Can you work these out from the model? Positions are in its coordinate system, mm. A direction names the side the tool comes from. Round coordinates to 2 decimals unless told otherwise and drop trailing zeros. Loops run counter-clockwise (first coordinate to the right, second up) from the corner with the lowest first, then second, coordinate; pieces in that order, holes last. Notation, with made-up numbers: (-19.5, -25.5) -> (-9.5, -25.5) arc R19 ccw to (-9.5, -21.5) -> close; hole circle Ø7 at (36.25, 80.5). An arc over 180 degrees is marked (long way). Use a Markdown table: item, result.
from build123d import *

# Parameters (mm, degrees)
SKETCH1_R           = 60
BOSS_EXTRUDE1_DEPTH = 10
SKETCH2_R           = 60
SKETCH2_R_2         = 55
BOSS_EXTRUDE2_DEPTH = 20
SKETCH3_R           = 12.5
CUT_EXTRUDE1_DEPTH  = 11


with BuildPart() as part:
    # Sketch1 → Boss-Extrude1 (new body)
    with BuildSketch(Plane(origin=(0, 0, 0), x_dir=(0, 0, -1), z_dir=(1, 0, 0))):
        Circle(SKETCH1_R)
    extrude(amount=BOSS_EXTRUDE1_DEPTH)

    # Sketch2 → Boss-Extrude2 (add)
    with BuildSketch(Plane(origin=(10, 0, 0), x_dir=(0, 0, -1), z_dir=(1, 0, 0))):
        Circle(SKETCH2_R)
        Circle(SKETCH2_R_2, mode=Mode.SUBTRACT)
    extrude(amount=BOSS_EXTRUDE2_DEPTH)

    # Sketch3 → Cut-Extrude1 (cut, through all)
    with BuildSketch(Plane(origin=(10, 0, 0), x_dir=(0, 0, -1), z_dir=(1, 0, 0))):
        Circle(SKETCH3_R)
    extrude(amount=-CUT_EXTRUDE1_DEPTH, mode=Mode.SUBTRACT)


solid = part.part
1. I want a section at C-C (x = 22.5). Please give me the cut outline in (y, z), plus the area to 3 significant figures.
Answer sheet:
| item | result |
|---|---|
| outline | circle Ø120 at (0, 0); hole circle Ø110 at (0, 0) |
| area | 1,810 mm² |
2. If we mould it in two halves opening along Y, with no side actions, what happens to faces 3 (the cylindrical face through (5.07, 3.755, -11.923)), 4 (the cylindrical face through (19.86, -53.692, 11.923)), 5 (the flat face through (30, -49, -26)), 6 (the cylindrical face through (14.79, 2.64, 59.94))? For each: +Y half, -Y half, draft (parallel to the pull), parting line (faces both ways), or undercut.
Answer sheet:
| item | result |
|---|---|
| face 3 | undercut |
| face 4 | undercut |
| face 5 | draft |
| face 6 | parting line |
3. I want a section at D-D (z = 32.5). Please give me the cut outline in (x, y).
Answer sheet:
| item | result |
|---|---|
| outline | (0, -50.44) -> (30, -50.44) -> (30, -44.37) -> (10, -44.37) -> (10, 44.37) -> (30, 44.37) -> (30, 50.44) -> (0, 50.44) -> close |
4. Will these pins go through, and if not, where does the flat tip stop? pin 1 Ø3 at (x, y) = (24.5, -3) entering from -Z; pin 2 Ø1.5 at (x, z) = (23, -33.5) entering from -Y; pin 3 Ø1 at (x, z) = (19.5, 2) entering from +Y.
Answer sheet:
| item | result |
|---|---|
| pin 1 | stops at z = -59.98 |
| pin 2 | stops at y = -50.27 |
| pin 3 | stops at y = 59.98 |
5. I want a section at A-A (z = 0). Please give me the cut outline in (x, y), plus the area to 3 significant figures.
Answer sheet:
| item | result |
|---|---|
| outline | (0, -60) -> (30, -60) -> (30, -55) -> (10, -55) -> (10, -12.5) -> (0, -12.5) -> close; (0, 12.5) -> (10, 12.5) -> (10, 55) -> (30, 55) -> (30, 60) -> (0, 60) -> close |
| area | 1,150 mm² |
6. Which directions (+Z, -Z, +X, -X, +Y, -Y) give clear straight access to the entire face, cutting with the end or side of a thin tool? Please do faces 1 (the flat face through (0, 14, 1)), 2 (the flat face through (10, 13, 1)).
Answer sheet:
| item | result |
|---|---|
| face 1 | +Z, -Z, -X, +Y, -Y |
| face 2 | +X |
7. I need wall thicknesses on line 1 (Y direction, x = 2.75, z = 0); line 2 (X direction, y = -36, z = -34); line 3 (Z direction, x = 25.25, y = 1). Which ranges of each line are inside material? Lowest first, please.
Answer sheet:
| item | result |
|---|---|
| line 1 | y = -60 to -12.5, 12.5 to 60 |
| line 2 | x = 0 to 10 |
| line 3 | z = -59.99 to -54.99, 54.99 to 59.99 |
